Read the model definition and answer for the solid it produces. Units are mm, in the model's axes. A direction names the side the tool comes from. Coordinates: 2 decimals unless noted, no trailing zeros. Write each loop counter-clockwise with the first axis right and the second up, starting at its lowest first coordinate (ties: lowest second). Pieces come first, ordered by that corner, then holes. Notation, with made-up numbers: (7.5, -6.5) -> (45.5, -6.5) arc R26 ccw to (45.5, 10.5) -> close; hole circle Ø9 at (-4.5, 42.25). An arc over 180 degrees is marked (long way). Use CSV: the item, a comma, the result in double quotes.
from build123d import *

# Parameters (mm, degrees)
ESQUISSE1_R                               = 14
BOSS_EXTRU_1_DEPTH                        = 150
CHANFREIN1_SIZE                           = 1
DIAM_TRE_DU_PER_AGE_14_0_14_1_D           = 14
DIAM_TRE_DU_PER_AGE_14_0_14_1_DEPTH       = 35
DIAM_TRE_DU_PER_AGE_14_0_14_1_CSINK_D     = 15
DIAM_TRE_DU_PER_AGE_14_0_14_1_CSINK_ANGLE = 90
DIAM_TRE_DU_PER_AGE_14_0_14_1_TIP         = 4.206024333
CHANFREIN2_SIZE                           = 0.5
TROU_TARAUD_M8X1_01_D                     = 7
TROU_TARAUD_M8X1_01_DEPTH                 = 25
TROU_TARAUD_M8X1_01_TIP                   = 2.103012167


with BuildPart() as part:
    # Esquisse1 → Boss.-Extru.1 (new body)
    with BuildSketch(Plane(origin=(0, 0, 0), x_dir=(1, 0, 0), z_dir=(0, 1, 0))):
        with Locations(Location((0, 0, 0), (0, 0, 270))):  # turned: the seam where the file's is
            Circle(ESQUISSE1_R)
    extrude(amount=BOSS_EXTRU_1_DEPTH)

    # Chanfrein1
    chanfrein1_edges = [part.edges().sort_by_distance(p)[0] for p in [
        (0, 150, -14),
    ]]
    chamfer(chanfrein1_edges, length=CHANFREIN1_SIZE)

    # Diamètre du perçage Ø14.0 (14)1
    with Locations(Plane(origin=(0, 150, 0), x_dir=(-1, 0, 0), z_dir=(0, 1, 0))):
        with Locations((0, 0)):
            CounterSinkHole(DIAM_TRE_DU_PER_AGE_14_0_14_1_D / 2, DIAM_TRE_DU_PER_AGE_14_0_14_1_CSINK_D / 2, depth=DIAM_TRE_DU_PER_AGE_14_0_14_1_DEPTH, counter_sink_angle=DIAM_TRE_DU_PER_AGE_14_0_14_1_CSINK_ANGLE)
            with Locations((0, 0, -(DIAM_TRE_DU_PER_AGE_14_0_14_1_DEPTH + DIAM_TRE_DU_PER_AGE_14_0_14_1_TIP / 2))):  # 118° drill point
                Cone(0, DIAM_TRE_DU_PER_AGE_14_0_14_1_D / 2, DIAM_TRE_DU_PER_AGE_14_0_14_1_TIP, mode=Mode.SUBTRACT)

    # Chanfrein2
    chanfrein2_edges = [part.edges().sort_by_distance(p)[0] for p in [
        (0, 0, -14),
    ]]
    chamfer(chanfrein2_edges, length=CHANFREIN2_SIZE)

    # Trou taraudé M8x1.01
    with Locations(Plane.XZ):
        with Locations((0, 0)):
            Hole(TROU_TARAUD_M8X1_01_D / 2, depth=TROU_TARAUD_M8X1_01_DEPTH)
            with Locations((0, 0, -(TROU_TARAUD_M8X1_01_DEPTH + TROU_TARAUD_M8X1_01_TIP / 2))):  # 118° drill point
                Cone(0, TROU_TARAUD_M8X1_01_D / 2, TROU_TARAUD_M8X1_01_TIP, mode=Mode.SUBTRACT)

    # Esquisse11 → Trou taraudé M42 (revolve, cut)
    with BuildSketch(Plane(origin=(0, 140, 0), x_dir=(0, 1, 0), z_dir=(1, 0, 0))):
        Polygon((0, 0), (0, 14), (2.25, 14), (1.65, 13.4), (1.65, 0), align=None)
    revolve(axis=Axis((0, 140, -6.35), (0, 0, 1)), mode=Mode.SUBTRACT)


solid = part.part
1. A cutting plane is placed at B-B (y = 101). Give the vertices of the cut face in (x, z).
Solutions:
outline,"circle Ø28 at (0, 0)"
2. Each of these flat-tipped pins is pushed along its axis until it touches: pin 1 Ø5.5 at (x, z) = (0, 0) entering from -Y; pin 2 Ø8 at (x, y) = (1, 31) entering from -Z; pin 3 Ø6 at (y, z) = (19, 10) entering from +X; pin 4 Ø12 at (x, y) = (-10.5, 46) entering from +Z. Where does it stop, or does it pass through?
Solutions:
pin 1,"stops at y = 25.45"
pin 2,"stops at z = -14"
pin 3,"stops at x = 12.12"
pin 4,"stops at z = 13.26"
3. Find the intervals of material crossed by line 1 along X through (y, z) = (6.75, 0); line 2 along Y through (x, z) = (0, 10); line 3 along X through (y, z) = (124.5, 0), in increasing order.
Solutions:
line 1,"x = -14 to -3.5, 3.5 to 14"
line 2,"y = 0 to 138.35, 141.65 to 150"
line 3,"x = -14 to -7, 7 to 14"
4. For a pull along X with two mould halves and no side action, classify faces 1 (the cylindrical face through (-0.496, 141.574, 10.055)), 2 (the flat face through (-6, 150, 6)), 3 (the cylindrical face through (-13.67, 73.71, -3.03)) as pulls with the +X half, pulls with the -X half, needs draft (parallel to the pull), parting line crosses it, or undercut.
Solutions:
face 1,"undercut"
face 2,"needs draft"
face 3,"parting line crosses it"
5. A cutting plane is placed at A-A (y = 140). Give the vertices of the cut face in (x, z), and give its area (3 significant figures).
Solutions:
outline,"(-2.09, 13.84) arc R14 ccw (long way) to (2.09, 13.84) -> (1.65, 13.4) -> (1.65, 6.8) arc R7 cw (long way) to (-1.65, 6.8) -> (-1.65, 13.4) -> close"
area,"438 mm^2"
6. A tool of negligible diameter and unlimited length cuts with its end or side. For faces 4 (the cylindrical face through (-3.233, 12.675, -1.341)), 5 (the cylindrical face through (-1.517, 132.008, -6.834)), 6 (the flat face through (-3, 0, 3)), from which of +Z, -Z, +X, -X, +Y, -Y can it reach the whole face along a straight path? Write none if from no direction.
Solutions:
face 4,"-Y"
face 5,"+Y"
face 6,"+Z, -Z, +X, -X, -Y"
